```python
from build123d import *

# Parameters (mm, degrees)
SKETCH1_R           = 2.55
BOSS_EXTRUDE2_DEPTH = 6
FILLET1_R           = 2.5
SKETCH3_R           = 7.975
CUT_EXTRUDE2_DEPTH  = 47.561319795
SKETCH2_R           = 1.25
CUT_EXTRUDE1_DEPTH  = 47.561319795
SKETCH6_W           = 40
SKETCH6_H           = 50
CUT_EXTRUDE5_DEPTH  = 1


with BuildPart() as part:
    # Sketch1 → Boss-Extrude2 (new body)
    with BuildSketch(Plane.XY):
        with BuildLine():
            Line((-10, -15), (-10, 5))
            Line((-10, 5), (-14, 30))
            ThreePointArc((-14, 30), (0, 44), (14, 30))
            Line((14, 30), (10, 5))
            Line((10, 5), (10, -15))
            Line((10, -15), (-10, -15))
        make_face()
        Circle(SKETCH1_R, mode=Mode.SUBTRACT)
        with Locations((0, -10)):
            Circle(SKETCH1_R, mode=Mode.SUBTRACT)
    extrude(amount=BOSS_EXTRUDE2_DEPTH)

    # Fillet1
    fillet1_edges = [part.edges().sort_by_distance(p)[0] for p in [
        (14, 30, 3),
        (10, 5, 3),
        (10, -15, 3),
        (-10, -15, 3),
        (-10, 5, 3),
        (-14, 30, 3),
    ]]
    fillet(fillet1_edges, radius=FILLET1_R)

    # Sketch3 → Cut-Extrude2 (cut, through all)
    with BuildSketch(Plane.XY.offset(6)):
        with Locations((0, 30)):
            Circle(SKETCH3_R)
    extrude(amount=-CUT_EXTRUDE2_DEPTH, mode=Mode.SUBTRACT)

    # Sketch2 → Cut-Extrude1 (cut, through all)
    with BuildSketch(Plane.XY.offset(6)):
        with Locations((-9, 24.5)):
            Circle(SKETCH2_R)
        with Locations((9, 24.5)):
            Circle(SKETCH2_R)
        with Locations((-9, 35.5)):
            Circle(SKETCH2_R)
        with Locations((9, 35.5)):
            Circle(SKETCH2_R)
    extrude(amount=-CUT_EXTRUDE1_DEPTH, mode=Mode.SUBTRACT)

    # Sketch6 → Cut-Extrude5 (cut)
    with BuildSketch(Plane.XY.offset(6)):
        with Locations((0, 30)):
            Rectangle(SKETCH6_W, SKETCH6_H)
    extrude(amount=-CUT_EXTRUDE5_DEPTH, mode=Mode.SUBTRACT)


solid = part.part
```
Geometry: final body of the model. Coordinates: model frame, mm. A direction names the side the tool comes from. Give positions to 0.01 mm unless a question says otherwise; leave off trailing zeros. Order: outer loops, then holes, each group sorted by start corner. A loop starts at its lowest first (then second) coordinate and runs counter-clockwise, first axis right, second up. Notation, with made-up numbers: M -18.75,5 L 30.25,5 A23 cw 30.25,33 Z; hole C -29.5,74 d6. An arc over 180 degrees is marked long. Answer as CSV lines item,"result". Start each with the question number.
1) Line query: line 1 (Y direction, x = -9, z = 1.2); line 2 (Y direction, x = 2.25, z = 2.5); line 3 (Y direction, x = 2, z = 1.45). Output: solid intervals per line, ascending. Write a range as from..to.
2) Mould query, pull axis Y, two halves, no side actions, for faces 1 (the cylindrical face through (3.68, 22.925, 2.535)), 2 (the flat face through (0, -5, 6)), 3 (the flat face through (-0.1, 5, 5.5)). Classes: +Y half, -Y half, draft (parallel to the pull), parting line (faces both ways), or undercut.
3) Cut plane B-B (y = -10). Output: boundary loops of the cut face in (x, z), then the cut area to 3 significant figures.
4) Cut plane D-D (x = -9). Output: boundary loops of the cut face in (y, z).
5) Cut plane A-A (z = 2.05). Output: boundary loops of the cut face in (x, y) (3 decimals), then the cut area to 3 significant figures.
6) Set-up query: faces 4 (the flat face through (0, 20, 5)), 5 (the flat face through (10, -4, 3)), 6 (the flat face through (-10, -4, 3)). Return all of +Z, -Z, +X, -X, +Y, -Y with unobstructed straight access to the full face (end or side cutting, diameter ignored); none if empty.
7) Cut plane C-C (x = 0). Output: boundary loops of the cut face in (y, z) (3 decimals).
8) First-contact query: P1, Ø4, axis at x = 9, y = 24.5, coming from the +Z side; P2, Ø1.5, axis at x = -1.5, z = 0.5, coming from the +Y side; P3, Ø0.8, axis at x = 0.5, z = 5.5, coming from the +Y side. Flat tips, straight axial feed; report the tip coordinate or a pass-through.
Findings below:
1,line 1,"y = -14.5..23.25, 25.75..34.25, 36.75..40.72"
1,line 2,"y = -15..-11.2, -8.8..-1.2, 1.2..22.35, 37.65..43.82"
1,line 3,"y = -15..-11.58, -8.42..-1.58, 1.58..22.28, 37.72..43.86"
2,face 1,"undercut"
2,face 2,"draft"
2,face 3,"+Y half"
3,outline,"M -10,0 L -2.55,0 L -2.55,6 L -10,6 Z; M 2.55,0 L 10,0 L 10,6 L 2.55,6 Z"
3,area,"89.4 mm²"
4,outline,"M -14.5,0 L 23.25,0 L 23.25,5 L 5,5 L 5,6 L -14.5,6 Z; M 25.75,0 L 34.25,0 L 34.25,5 L 25.75,5 Z; M 36.75,0 L 40.72,0 L 40.72,5 L 36.75,5 Z"
5,outline,"M -13.998,30.23 A2.5 ccw -13.967,29.794 L -10.031,5.196 A2.5 cw -10,4.801 L -10,-12.5 A2.5 ccw -7.5,-15 L 7.5,-15 A2.5 ccw 10,-12.5 L 10,4.801 A2.5 cw 10.031,5.196 L 13.967,29.794 A2.5 ccw 13.998,30.23 A14 ccw Z; hole C -9,24.5 d2.5; hole C -9,35.5 d2.5; hole C 0,30 d15.95; hole C 0,-10 d5.1; hole C 0,0 d5.1; hole C 9,24.5 d2.5; hole C 9,35.5 d2.5"
5,area,"1,040 mm²"
6,face 4,"+Z, +X, -X, +Y"
6,face 5,"+Z, -Z, +X, -Y"
6,face 6,"+Z, -Z, -X, -Y"
7,outline,"M -15,0 L -12.55,0 L -12.55,6 L -15,6 Z; M -7.45,0 L -2.55,0 L -2.55,6 L -7.45,6 Z; M 2.55,0 L 22.025,0 L 22.025,5 L 5,5 L 5,6 L 2.55,6 Z; M 37.975,0 L 44,0 L 44,5 L 37.975,5 Z"
8,P1,"stops at z = 5"
8,P2,"stops at y = 43.98"
8,P3,"stops at y = 5"
